from build123d import *

# Parameters (mm, degrees)
BOSS_EXTRUDE1_START  = 406.4
SKETCH2_W            = 406.4
SKETCH2_H            = 457.2
BOSS_EXTRUDE1_DEPTH  = 25.4
SKETCH5_W            = 406.4
SKETCH5_H            = 38.1
BOSS_EXTRUDE2_DEPTH  = 431.8
BOSS_EXTRUDE3_DEPTH  = 406.4
BOSS_EXTRUDE5_DEPTH  = 406.4
BOSS_EXTRUDE6_DEPTH  = 406.4
BOSS_EXTRUDE8_START  = -25.4
BOSS_EXTRUDE8_DEPTH  = 355.6
BOSS_EXTRUDE10_DEPTH = 12.7


with BuildPart() as part:
    # Sketch2 → Boss-Extrude1 (new body)
    with BuildSketch(Plane(origin=(0, 0, 0), x_dir=(1, 0, 0), z_dir=(0, 1, 0)).offset(BOSS_EXTRUDE1_START)):
        Rectangle(SKETCH2_W, SKETCH2_H)
    extrude(amount=BOSS_EXTRUDE1_DEPTH)

    # Sketch5 → Boss-Extrude2 (add)
    with BuildSketch(Plane(origin=(0, 431.8, 0), x_dir=(1, 0, 0), z_dir=(0, 1, 0))):
        with Locations((0, 209.55)):
            Rectangle(SKETCH5_W, SKETCH5_H)
    extrude(amount=BOSS_EXTRUDE2_DEPTH)

    # Sketch6 → Boss-Extrude3 (add)
    with BuildSketch(Plane(origin=(203.2, 0, 0), x_dir=(0, 0, -1), z_dir=(1, 0, 0))):
        with BuildLine():
            Line((190.5, 431.8), (228.6, 431.8))
            Line((228.6, 431.8), (228.6, 863.6))
            Line((228.6, 863.6), (209.55, 863.6))
            ThreePointArc((209.55, 863.6), (178.726471845, 648.639640948), (190.5, 431.8))
        make_face()
    extrude(amount=-BOSS_EXTRUDE3_DEPTH)

    # Sketch7 → Boss-Extrude5 (add)
    with BuildSketch(Plane(origin=(203.2, 0, 0), x_dir=(0, 0, -1), z_dir=(1, 0, 0))):
        with BuildLine():
            Line((-228.6, 431.8), (-228.6, 406.4))
            Line((-228.6, 406.4), (190.5, 406.4))
            Line((190.5, 406.4), (190.5, 431.8))
            ThreePointArc((190.5, 431.8), (-19.05, 439.760210116), (-228.6, 431.8))
        make_face()
    extrude(amount=-BOSS_EXTRUDE5_DEPTH)

    # Sketch8 → Boss-Extrude6 (add)
    with BuildSketch(Plane(origin=(203.2, 0, 0), x_dir=(0, 0, -1), z_dir=(1, 0, 0))):
        with BuildLine():
            Line((190.5, 863.6), (228.6, 863.6))
            Line((228.6, 863.6), (228.6, 767.986138045))
            Line((228.6, 767.986138045), (190.5, 767.986138045))
            ThreePointArc((190.5, 767.986138045), (183.89577559, 815.793069023), (190.5, 863.6))
        make_face()
    extrude(amount=-BOSS_EXTRUDE6_DEPTH)

    # Sketch9 → Boss-Extrude8 (add)
    with BuildSketch(Plane(origin=(203.2, 0, 0), x_dir=(0, 0, -1), z_dir=(1, 0, 0)).offset(BOSS_EXTRUDE8_START)):
        with BuildLine():
            Line((190.064521118, 864.483944692), (224.793246745, 864.483944692))
            Line((224.793246745, 864.483944692), (224.793246745, 863.6))
            Line((224.793246745, 863.6), (224.793246745, 408.97647982))
            Line((224.793246745, 408.97647982), (-229.126005902, 408.97647982))
            Line((-229.126005902, 408.97647982), (-229.126005902, 432.005066032))
            ThreePointArc((-229.126005902, 432.005066032), (-19.530742392, 440.435933777), (190.064521118, 432.005066032))
            ThreePointArc((190.064521118, 432.005066032), (177.09008034, 600.056508721), (190.064521118, 768.10795141))
            ThreePointArc((190.064521118, 768.10795141), (183.373440165, 816.295948051), (190.064521118, 864.483944692))
        make_face()
    extrude(amount=-BOSS_EXTRUDE8_DEPTH)

    # Sketch11 → Boss-Extrude10 (add)
    with BuildSketch(Plane.XZ.offset(-406.4)):
        Polygon((0, 0), (0, 1.931960206), (-1.331020628, 0), align=None)
    extrude(amount=BOSS_EXTRUDE10_DEPTH)


solid = part.part
Build history of the part. All positions in model axes, mm. A direction names the side the tool comes from. Give positions to 0.01 mm unless a question says otherwise; leave off trailing zeros. Loops run counter-clockwise (first coordinate to the right, second up) from the corner with the lowest first, then second, coordinate; pieces in that order, holes last. Notation, with made-up numbers: (-1.5, 18.25) -> (43.5, 18.25) arc R9 ccw to (43.5, 34.25) -> close; hole circle Ø2 at (53, 14). An arc over 180 degrees is marked (long way). Answer in a Markdown table with one row per item.
Item 1: Slice it at A-A on x = -71. Write the cut outline in (y, z), plus the area to 3 significant figures.
Findings below:
| item | result |
|---|---|
| outline | (406.4, -228.6) -> (863.6, -228.6) -> (863.6, -224.79) -> (864.48, -224.79) -> (864.48, -190.06) arc R176.87 ccw to (768.11, -190.06) arc R1094.83 ccw to (432.01, -190.06) arc R2609.53 ccw to (432.01, 229.13) -> (408.98, 229.13) -> (408.98, 228.6) -> (406.4, 228.6) -> close |
| area | 34,100 mm² |
Item 2: Tool access for faces 4 (the flat face through (-203.2, 549, -185)), 5 (the cylindrical face through (-190.322, 815.115, -183.897)), 6 (the flat face through (-0.9, 408.7, 228.6)): list every direction of +Z, -Z, +X, -X, +Y, -Y with a clear straight run to the whole face (end or side of a thin tool).
Findings below:
| item | result |
|---|---|
| face 4 | +Z, -Z, -X, +Y, -Y |
| face 5 | +Z, -X |
| face 6 | +Z, -Y |
Item 3: Slice it at B-B on z = 13. Write the cut outline in (x, y), plus the area to 3 significant figures.
Findings below:
| item | result |
|---|---|
| outline | (-203.2, 406.4) -> (203.2, 406.4) -> (203.2, 439.75) -> (177.8, 439.75) -> (177.8, 440.43) -> (-177.8, 440.43) -> (-177.8, 439.75) -> (-203.2, 439.75) -> close |
| area | 13,800 mm² |
Item 4: Probe line 1 along Z through (x, y) = (-109, 642); line 2 along Y through (x, z) = (180, 21); line 3 along Y through (x, z) = (-152.5, 2). List the from-to ranges inside material, lowest first. Write a range as [from, to].
Findings below:
| item | result |
|---|---|
| line 1 | z = [-228.6, -177.89] |
| line 2 | y = [406.4, 439.76] |
| line 3 | y = [406.4, 440.38] |
Item 5: Mould opens along Z. For faces 1 (the flat face through (-3, 632, -228.6)), 2 (the cylindrical face through (2.489, 440.434, 22.468)), 3 (the cylindrical face through (190.678, 815.115, -183.897)) say: pulls with the +Z half, pulls with the -Z half, needs draft (parallel to the pull), parting line crosses it, or undercut.
Findings below:
| item | result |
|---|---|
| face 1 | pulls with the -Z half |
| face 2 | undercut |
| face 3 | pulls with the +Z half |
Item 6: Slice it at C-C on y = 567. Write the cut outline in (x, z), plus the area to 3 significant figures.
Findings below:
| item | result |
|---|---|
| outline | (-203.2, -228.6) -> (203.2, -228.6) -> (203.2, -178.14) -> (177.8, -178.14) -> (177.8, -177.59) -> (-177.8, -177.59) -> (-177.8, -178.14) -> (-203.2, -178.14) -> close |
| area | 20,700 mm² |
Item 7: Flat gauge pins, fed straight in: P1, Ø1, axis at x = -4, y = 864, coming from the -Z side; P2, Ø6, axis at x = 149, z = -117, coming from the -Y side; P3, Ø1, axis at y = 399, z = 0.5, coming from the +X side; P4, Ø1.5, axis at x = -0.5, y = 399, coming from the -Z side. Where does each tip first touch, or does it go through?
Findings below:
| item | result |
|---|---|
| P1 | stops at z = -228.6 |
| P2 | stops at y = 406.4 |
| P3 | stops at x = 0 |
| P4 | stops at z = 0 |
